Geometry: see drawing. Coordinates: mm, zero at the bounding-box minimum. Give positions to 0.01 mm unless a question says otherwise; leave off trailing zeros. Write each loop counter-clockwise with the first axis right and the second up, starting at its lowest first coordinate (ties: lowest second). Pieces come first, ordered by that corner, then holes. Notation, with made-up numbers: (59, 54.25) -> (113, 54.25) arc R23 cw to (113, 64.25) -> close; hole circle Ø11 at (78.5, 5). An arc over 180 degrees is marked (long way). Use CSV: the item, a comma, the result in double quotes. Start each with the question number.
1) Material intervals for line 1 (X direction, y = 9, z = 1.2); line 2 (X direction, y = 8, z = 0.3); line 3 (Y direction, x = 9.5, z = 1.45), sorted ascending. Write a range as [from, to].
2) Section B-B (z = 1). Output: boundary loops of the cut face in (x, y).
3) Section A-A (y = 8). Output: boundary loops of the cut face in (x, z), plus the area to 3 significant figures.
4) Draft query along Y for the marked faces 1 and 2. Return one class per face: pulls with the +Y half, pulls with the -Y half, needs draft (parallel to the pull), parting line crosses it, or undercut.
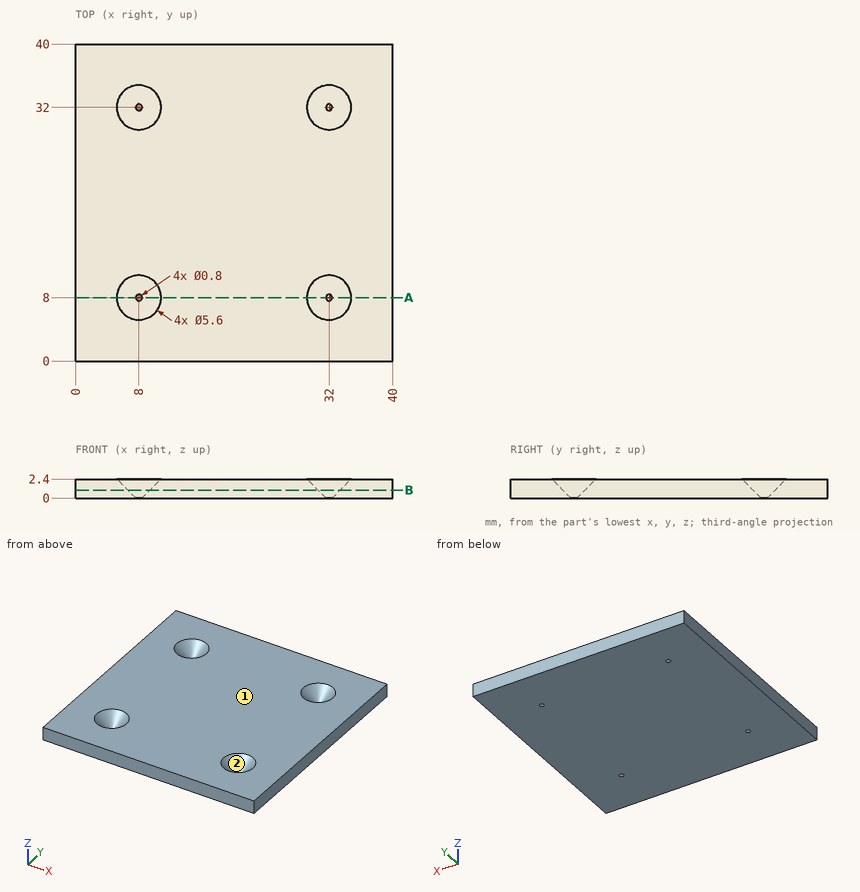
Answers follow:
1,line 1,"x = [0, 6.75], [9.25, 30.75], [33.25, 40]"
1,line 2,"x = [0, 7.3], [8.7, 31.3], [32.7, 40]"
1,line 3,"y = [0, 6.92], [9.08, 30.92], [33.08, 40]"
2,outline,"(0, 0) -> (40, 0) -> (40, 40) -> (0, 40) -> close; hole circle Ø2.8 at (8, 8); hole circle Ø2.8 at (8, 32); hole circle Ø2.8 at (32, 8); hole circle Ø2.8 at (32, 32)"
3,outline,"(0, 0) -> (7.6, 0) -> (5.2, 2.4) -> (0, 2.4) -> close; (8.4, 0) -> (31.6, 0) -> (29.2, 2.4) -> (10.8, 2.4) -> close; (32.4, 0) -> (40, 0) -> (40, 2.4) -> (34.8, 2.4) -> close"
3,area,"80.6 mm^2"
4,face 1,"needs draft"
4,face 2,"undercut"
